Read the model definition and answer for the solid it produces. Units are mm, in the model's axes. A direction names the side the tool comes from. Coordinates: 2 decimals unless noted, no trailing zeros. Order: outer loops, then holes, each group sorted by start corner. A loop starts at its lowest first (then second) coordinate and runs counter-clockwise, first axis right, second up. Notation, with made-up numbers: M 50.5,48 L 92.5,48 A22 cw 92.5,74 Z; hole C 85.5,59.5 d9. An arc over 180 degrees is marked long. Write each question's results on one line, items separated by ' | '.
```python
from build123d import *

# Parameters (mm, degrees)
PAD_DEPTH       = 25
SKETCH001_R     = 4.3
POCKET_DEPTH    = 60.801
SKETCH002_R     = 3.3
POCKET001_DEPTH = 60.801
FILLET_R        = 4
FILLET001_R     = 2
SKETCH003_R     = 6.75
POCKET002_DEPTH = 5
SKETCH004_R     = 6.75
POCKET003_DEPTH = 5
SKETCH005_R     = 5.25
POCKET004_DEPTH = 5
POCKET005_DEPTH = 4


with BuildPart() as part:
    # Sketch → Pad (new body)
    with BuildSketch(Plane.XZ):
        Polygon((-72.5, -30.4), (72.5, -30.4), (72.5, -20.4), (39.6, -20.4), (39.6, 20.4), (72.5, 20.4), (72.5, 30.4), (-72.5, 30.4), (-72.5, 20.4), (-39.6, 20.4), (-39.6, -20.4), (-72.5, -20.4), align=None)
        Polygon((-30.4, -20.9), (-30.4, 12.4), (-17.4, 12.4), (-17.4, 22.9), (17.4, 22.9), (17.4, 12.4), (30.4, 12.4), (30.4, -20.9), align=None, mode=Mode.SUBTRACT)
    extrude(amount=PAD_DEPTH)

    # Sketch001 (on Face7 of Pad) → Pocket (cut, through all)
    with BuildSketch(Plane(origin=(0, 0, 30.4), x_dir=(-1, 0, 0), z_dir=(0, 0, 1))):
        with Locations((-60, 12.5)):
            Circle(SKETCH001_R)
        with Locations((60, 12.5)):
            Circle(SKETCH001_R)
    extrude(amount=-POCKET_DEPTH, mode=Mode.SUBTRACT)

    # Sketch002 (on Face13 of Pocket) → Pocket001 (cut, through all)
    with BuildSketch(Plane(origin=(0, 0, 30.4), x_dir=(-1, 0, 0), z_dir=(0, 0, 1))):
        with Locations((-23, 6)):
            Circle(SKETCH002_R)
        with Locations((-23, 19)):
            Circle(SKETCH002_R)
        with Locations((23, 19)):
            Circle(SKETCH002_R)
        with Locations((23, 6)):
            Circle(SKETCH002_R)
    extrude(amount=-POCKET001_DEPTH, mode=Mode.SUBTRACT)

    # Fillet
    fillet_edges = [part.edges().sort_by_distance(p)[0] for p in [
        (-72.5, -25, 25.4),
        (-72.5, -25, -25.4),
        (72.5, -25, -25.4),
        (72.5, -25, 25.4),
        (-72.5, 0, 25.4),
        (-72.5, 0, -25.4),
        (72.5, 0, -25.4),
        (72.5, 0, 25.4),
    ]]
    fillet(fillet_edges, radius=FILLET_R)

    # Fillet001
    fillet001_edges = [part.edges().sort_by_distance(p)[0] for p in [
        (-39.6, -12.5, -20.4),
        (-39.6, -12.5, 20.4),
        (39.6, -12.5, 20.4),
        (39.6, -12.5, -20.4),
    ]]
    fillet(fillet001_edges, radius=FILLET001_R)

    # Sketch003 (on Face13 of Fillet001) → Pocket002 (cut)
    with BuildSketch(Plane(origin=(0, 0, 30.4), x_dir=(-1, 0, 0), z_dir=(0, 0, 1))):
        with Locations((-60, 12.5)):
            Circle(SKETCH003_R)
        with Locations((60, 12.5)):
            Circle(SKETCH003_R)
    extrude(amount=-POCKET002_DEPTH, mode=Mode.SUBTRACT)

    # Sketch004 (on Face13 of Pocket002) → Pocket003 (cut)
    with BuildSketch(Plane(origin=(0, 0, -30.4), x_dir=(-1, 0, 0), z_dir=(0, 0, 1))):
        with Locations((-60, 12.5)):
            Circle(SKETCH004_R)
        with Locations((60, 12.5)):
            Circle(SKETCH004_R)
    extrude(amount=POCKET003_DEPTH, mode=Mode.SUBTRACT)

    # Sketch005 (on Face13 of Pocket003) → Pocket004 (cut)
    with BuildSketch(Plane(origin=(0, 0, 30.4), x_dir=(-1, 0, 0), z_dir=(0, 0, 1))):
        with Locations((-23, 19)):
            Circle(SKETCH005_R)
        with Locations((-23, 6)):
            Circle(SKETCH005_R)
        with Locations((23, 6)):
            Circle(SKETCH005_R)
        with Locations((23, 19)):
            Circle(SKETCH005_R)
    extrude(amount=-POCKET004_DEPTH, mode=Mode.SUBTRACT)

    # Sketch006 (on Face13 of Pocket004) → Pocket005 (cut)
    with BuildSketch(Plane(origin=(0, 0, -30.4), x_dir=(-1, 0, 0), z_dir=(0, 0, 1))):
        Polygon((-20.026646, 13.85), (-17.053292, 19), (-20.026646, 24.15), (-25.973354, 24.15), (-28.946708, 19), (-25.973354, 13.85), align=None)
        Polygon((-20.026646, 0.85), (-17.053292, 6), (-20.026646, 11.15), (-25.973354, 11.15), (-28.946708, 6), (-25.973354, 0.85), align=None)
        Polygon((25.973354, 13.85), (28.946708, 19), (25.973354, 24.15), (20.026646, 24.15), (17.053292, 19), (20.026646, 13.85), align=None)
        Polygon((25.973354, 0.85), (28.946708, 6), (25.973354, 11.15), (20.026646, 11.15), (17.053292, 6), (20.026646, 0.85), align=None)
    extrude(amount=POCKET005_DEPTH, mode=Mode.SUBTRACT)


solid = part.part
```
(1) The mould has two halves that part along Z. Classify faces 1 (the flat face through (-23, -0.85, -28)), 2 (the flat face through (20, -21, -26.4)), 3 (the flat face through (54, -12, -20.4)): pulls with the +Z half, pulls with the -Z half, needs draft (parallel to the pull), parting line crosses it, or undercut.
Conclusion:
face 1: needs draft | face 2: pulls with the -Z half | face 3: undercut
(2) The part is cut by section D-D, the plane x = 23. Count the separate pieces of the cut face and the enclosed holes in it, then the cut area to 3 significant figures.
Conclusion:
separate pieces: 6 | enclosed holes: 0 | area: 256 mm²
(3) The part is cut by section A-A, the plane x = -44. Write down the section's boundary in (y, z).
Conclusion:
outline: M -25,-30.4 L 0,-30.4 L 0,-20.4 L -25,-20.4 Z; M -25,20.4 L 0,20.4 L 0,30.4 L -25,30.4 Z
(4) Straight lines are drawn through the part: line 1 (Y direction, x = 23, z = -23); line 2 (X direction, y = -12.5, z = 24); line 3 (X direction, y = -12.5, z = 22.1). For each, find the intervals that lie inside material, in ascending order.
Conclusion:
line 1: -25 to -22.3, -15.7 to -9.3, -2.7 to 0 | line 2: -72.5 to -64.3, -55.7 to 55.7, 64.3 to 72.5 | line 3: -72.5 to -64.3, -55.7 to -17.4, 17.4 to 55.7, 64.3 to 72.5
(5) Given pin 1 (6 mm diameter, centred on y = -7.5, z = -2.5, fed in from +X); pin 2 (9.5 mm diameter, centred on x = 23, y = -19, fed in from +Z); pin 3 (5 mm diameter, centred on y = -20.5, z = -13.5, fed in from -X), each flat-ended and moving along its own axis, determine where each tip first touches the part or whether it passes through.
Conclusion:
pin 1: x = 39.6 | pin 2: z = 25.4 | pin 3: x = -39.6
(6) The part is cut by section C-C, the plane x = 60. Write down the section's boundary in (y, z), then the cut area to 3 significant figures.
Conclusion:
outline: M -25,-30.4 L -19.25,-30.4 L -19.25,-25.4 L -16.8,-25.4 L -16.8,-20.4 L -25,-20.4 Z; M -25,20.4 L -16.8,20.4 L -16.8,25.4 L -19.25,25.4 L -19.25,30.4 L -25,30.4 Z; M -8.2,-25.4 L -5.75,-25.4 L -5.75,-30.4 L 0,-30.4 L 0,-20.4 L -8.2,-20.4 Z; M -8.2,20.4 L 0,20.4 L 0,30.4 L -5.75,30.4 L -5.75,25.4 L -8.2,25.4 Z | area: 279 mm²
(7) The part is cut by section B-B, the plane z = 5.5. Write down the section's boundary in (x, y).
Conclusion:
outline: M -39.6,-25 L -30.4,-25 L -30.4,0 L -39.6,0 Z; M 30.4,-25 L 39.6,-25 L 39.6,0 L 30.4,0 Z
(8) For faces 4 (the flat face through (60, -8, 25.4)), 5 (the flat face through (-24, -12, 12.4)), 6 (the cylindrical face through (71.297, -23.859, 25.47)), 7 (the flat face through (-18.52, -3.46, -28.43)), determine the directions among +Z, -Z, +X, -X, +Y, -Y from which every point of the face is accessible in a straight line to the end or side of a thin tool.
Conclusion:
face 4: +Z | face 5: +Y, -Y | face 6: +Z, -Z, +X, -Y | face 7: -Z
